from build123d import *

# Parameters (mm, degrees)
F0_R     = 15.875
F1_DEPTH = 850.9
F2_R     = 8.001
F3_DEPTH = 53.34
F4_R     = 2.0574
F5_DEPTH = 25.4
F6_R     = 15.875
F6_R_2   = 7.9883
F7_DEPTH = 50.8
F8_R     = 2.54
F9_DEPTH = 12.7


with BuildPart() as f1:
    # F0 (on Front) → F1 (new body)
    with BuildSketch(Plane.XZ):
        Circle(F0_R)
    extrude(amount=F1_DEPTH)

    # F2 (on face) → F3 (cut)
    with BuildSketch(Plane.XZ.offset(850.9)):
        Circle(F2_R)
    extrude(amount=-F3_DEPTH, mode=Mode.SUBTRACT)

    # F4 (on Right) → F5 (cut, symmetric)
    with BuildSketch(Plane.YZ):
        with Locations((-830.834, 0)):
            Circle(F4_R)
        with Locations((-20.066, 0)):
            Circle(F4_R)
    extrude(amount=F5_DEPTH, both=True, mode=Mode.SUBTRACT)

    # F6 (on face) → F7 (cut)
    with BuildSketch(Plane(origin=(0, 0, 0), x_dir=(-1, 0, 0), z_dir=(0, 1, 0))):
        Circle(F6_R)
        Circle(F6_R_2, mode=Mode.SUBTRACT)
    extrude(amount=-F7_DEPTH, mode=Mode.SUBTRACT)

    # F8 (on face) → F9 (cut)
    with BuildSketch(Plane(origin=(0, 0, 0), x_dir=(-1, 0, 0), z_dir=(0, 1, 0))):
        Circle(F8_R)
    extrude(amount=-F9_DEPTH, mode=Mode.SUBTRACT)


solid = f1.part
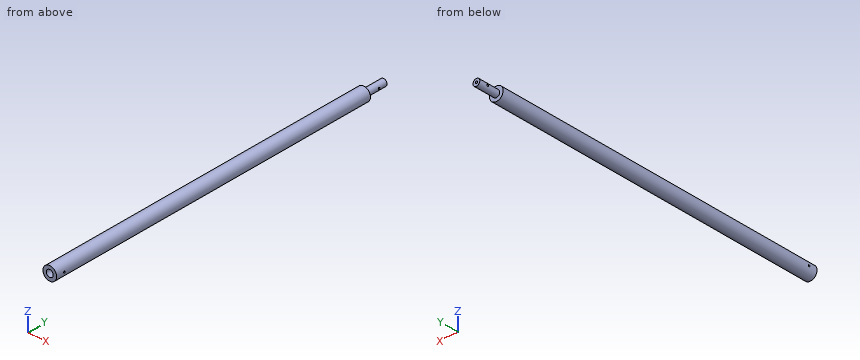
The model under review builds one solid part; all positions refer to its coordinate system, in mm. Give positions to 0.01 mm unless a question says otherwise; leave off trailing zeros. Write each loop counter-clockwise with the first axis right and the second up, starting at its lowest first coordinate (ties: lowest second). Pieces come first, ordered by that corner, then holes.
1. Wall thickness on L1, parallel to Y at x = -12, z = -3; L2, parallel to Y at x = 1.5, z = 1; L3, parallel to X at y = -539.5, z = -1: over which ranges is each line inside the solid? List them lowest first.
2. Add section A-A, the plane y = -589.5. Write out the cut boundary in (x, z) (3 decimals).
3. For P1, Ø3.5, axis at y = -830.834, z = 0, coming from the -X side; P2, Ø6, axis at x = -12, y = -536, coming from the +Z side; P3, Ø4.5, axis at x = 0, z = 0, coming from the +Y side; P4, Ø2, axis at x = 7.5, y = -393, coming from the -Z side, all flat-tipped, find the tip position at first contact; note any pin that passes through.
Worked answers:
1. L1: y = -850.9 to -50.8
1. L2: y = -797.56 to -21.86, -18.27 to -12.7
1. L3: x = -15.84 to 15.84
2. outline: circle Ø31.75 at (0, 0)
3. P1: passes through
3. P2: stops at z = 13.08
3. P3: stops at y = -12.7
3. P4: stops at z = -14.48
